```python
from build123d import *

# Parameters (mm, degrees)
SKETCH_1_R               = 20
EXTRUDE_1_DEPTH          = 10
SKETCH_2_R               = 12.5
EXTRUDE_2_DEPTH          = 8
SKETCH_3_R               = 4
CUT_EXTRUDE_1_DEPTH      = 19
EXTRUDE_3_DEPTH          = 10
PATTERN_CIRCULAR_1_COUNT = 40


with BuildPart() as part:
    # 草圖1 → 填料-伸長1 (new body)
    with BuildSketch(Plane.XY):
        Circle(SKETCH_1_R)
    extrude(amount=EXTRUDE_1_DEPTH)

    # 草圖2 → 填料-伸長2 (add)
    with BuildSketch(Plane.XY.offset(10)):
        Circle(SKETCH_2_R)
    extrude(amount=EXTRUDE_2_DEPTH)

    # 草圖3 → 除料-伸長1 (cut, through all)
    with BuildSketch(Plane.XY.offset(18)):
        Circle(SKETCH_3_R)
    extrude(amount=-CUT_EXTRUDE_1_DEPTH, mode=Mode.SUBTRACT)

    # 草圖4 → 填料-伸長3 (add)
    with BuildSketch(Plane(origin=(0, 0, 0), x_dir=(-1, 0, 0), z_dir=(0, 0, -1))):
        Polygon((-0.5, 21), (0.5, 21), (2, 16), (-2, 16), align=None)
    extrude_3 = extrude(amount=-EXTRUDE_3_DEPTH)

    # 環狀複製排列1: 填料-伸長3 ×40 about axis
    pattern_circular_1_axis = Axis((0, 0, 0), (0, 0, 1))
    for i in range(1, PATTERN_CIRCULAR_1_COUNT):
        add(extrude_3.rotate(pattern_circular_1_axis, i * 360 / PATTERN_CIRCULAR_1_COUNT))


solid = part.part
```
Check sheet for the modelled part. Datum: model origin and axes. Units: mm. A direction names the side the tool comes from. Give positions to 0.01 mm unless a question says otherwise; leave off trailing zeros. Write each loop counter-clockwise with the first axis right and the second up, starting at its lowest first coordinate (ties: lowest second). Pieces come first, ordered by that corner, then holes. Notation, with made-up numbers: (-27, 19) - (15, 19) arc R15 cw to (15, 43) - close; hole circle Ø7 at (74, 45). An arc over 180 degrees is marked (long way). Answer as a JSON object with one key per item and string values. Group by question number.
1) Sectioned sample at D-D (x = 10.5). Record the cut outline in (y, z).
2) Access from +Z, -Z, +X, -X, +Y, -Y to the whole of each face (thin tool, end or side, straight path). Record for faces 1 (the face through (20.14, 3.85, 4.93)), 2 (the face through (-0.65, 20.5, 4.93)), 3 (the face through (-19.94, -1.56, 4.93)).
3) Sectioned sample at A-A (y = 0). Record the cut outline in (x, z), then the cut area to 3 significant figures.
4) Depth check by flat-ended pin: P1, Ø3, axis at x = -2, z = 13.5, coming from the +Y side; P2, Ø1.5, axis at y = -2.5, z = 6.5, coming from the +X side; P3, Ø10, axis at x = -7.5, z = 6, coming from the +Y side. Enter the tip coordinate at first touch or a pass-through.
5) Sectioned sample at C-C (z = 12.75). Record the cut outline in (x, y), then the cut area to 3 significant figures.
6) Release check for a two-part mould opening along X. For faces 4 (the face through (1.56, -19.94, 4.93)), 5 (the face through (4.4, -0.4, 0)), 6 (the face through (-19.45, -4.66, 4.93)) record: pulls with the +X half, pulls with the -X half, needs draft (parallel to the pull), parting line crosses it, or undercut.
7) Thickness scan on probe 1 along Y at (x, z) = (0, 8.5); probe 2 along X at (y, z) = (15, 5.75); probe 3 along Y at (x, z) = (0, 14.25). Record the ranges inside material, lowest first. Write a range as from..to.
Geometry results:
{
 "1": {"outline": "(-17.02, 0) - (17.02, 0) - (17.02, 10) - (6.78, 10) - (6.78, 18) - (-6.78, 18) - (-6.78, 10) - (-17.02, 10) - close"},
 "2": {"face 1": "+Z, -Z, +X", "face 2": "+Z, -Z, +Y", "face 3": "+Z, -Z, -X"},
 "3": {"outline": "(-21, 0) - (-4, 0) - (-4, 18) - (-12.5, 18) - (-12.5, 10) - (-21, 10) - close; (4, 0) - (21, 0) - (21, 10) - (12.5, 10) - (12.5, 18) - (4, 18) - close", "area": "476 mm^2"},
 "4": {"P1": "stops at y = 12.49", "P2": "stops at x = 20.82", "P3": "stops at y = 20.82"},
 "5": {"outline": "circle Ø25 at (0, 0); hole circle Ø8 at (0, 0)", "area": "441 mm^2"},
 "6": {"face 4": "undercut", "face 5": "needs draft", "face 6": "pulls with the -X half"},
 "7": {"probe 1": "y = -21..-4, 4..21", "probe 2": "x = -14.7..-14.12, -13.23..13.23, 14.12..14.7", "probe 3": "y = -12.5..-4, 4..12.5"}
}
